For this review, take the finished solid that the model builds, in its own axes (mm). A direction names the side the tool comes from. Give positions to 0.01 mm unless a question says otherwise; leave off trailing zeros. Write each loop counter-clockwise with the first axis right and the second up, starting at its lowest first coordinate (ties: lowest second). Pieces come first, ordered by that corner, then holes. Notation, with made-up numbers: (-20.75, -4.5) -> (2.25, -4.5) arc R16 ccw to (2.25, 22.5) -> close; hole circle Ø7 at (-21, -38.5). An arc over 180 degrees is marked (long way). Write item = value, one per line.
```python
from build123d import *

# Parameters (mm, degrees)
F0_W     = 88
F0_H     = 30
F1_DEPTH = 5
F2_R     = 4
F3_DEPTH = 8
F4_R     = 4
F5_DEPTH = 8


with BuildPart() as f1:
    # F0 (on Front) → F1 (new body)
    with BuildSketch(Plane.XZ):
        Rectangle(F0_W, F0_H)
    extrude(amount=F1_DEPTH)

    # F2 (on face) → F3 (join)
    with BuildSketch(Plane.XZ.offset(5)):
        with Locations((-29, 0)):
            Circle(F2_R)
    extrude(amount=F3_DEPTH)

    # F4 (on face) → F5 (join)
    with BuildSketch(Plane.XZ.offset(5)):
        Circle(F4_R)
        with Locations((25, 0)):
            Circle(F4_R)
    extrude(amount=F5_DEPTH)


solid = f1.part
```
(1) To check wall thickness, follow probe 1 along Y at (x, z) = (3, 4.5); probe 2 along X at (y, z) = (-6, -3.5); probe 3 along X at (y, z) = (-6.75, 3). State the ranges of each line that lie inside material, in increasing order.
Answers below:
probe_1 = -5 to 0
probe_2 = -30.94 to -27.06, -1.94 to 1.94, 23.06 to 26.94
probe_3 = -31.65 to -26.35, -2.65 to 2.65, 22.35 to 27.65
(2) The part is to be moulded in two halves that separate along X. For faces 1 (the face through (-1, 0, 0)), 2 (the face through (-0.867, -8.944, -3.905)), 3 (the face through (-32.2, -8.9, -2.4)), 4 (the face through (-44, -2, 0)), say which applies: released by +X, released by -X, zero draft, split by the parting line, or undercut.
Answers below:
face_1 = zero draft
face_2 = undercut
face_3 = undercut
face_4 = released by -X
(3) Tool access review of faces 5 (the face through (-1, -2, 15)), 6 (the face through (-1, -5, 7)): name each direction out of +Z, -Z, +X, -X, +Y, -Y from which nothing blocks a thin tool from reaching the whole face with its end or side.
Answers below:
face_5 = +Z, +X, -X, +Y, -Y
face_6 = -Y
(4) Take a section at B-B (y = -8.75). Write out the cut boundary in (x, z).
Answers below:
outline = circle Ø8 at (-29, 0); circle Ø8 at (0, 0); circle Ø8 at (25, 0)
(5) Take a section at A-A (x = 0). Write out the cut boundary in (y, z), plus the area to 3 significant figures.
Answers below:
outline = (-13, -4) -> (-5, -4) -> (-5, -15) -> (0, -15) -> (0, 15) -> (-5, 15) -> (-5, 4) -> (-13, 4) -> close
area = 214 mm^2
(6) Take a section at C-C (z = 0). Write out the cut boundary in (x, y), plus the area to 3 significant figures.
Answers below:
outline = (-44, -5) -> (-33, -5) -> (-33, -13) -> (-25, -13) -> (-25, -5) -> (-4, -5) -> (-4, -13) -> (4, -13) -> (4, -5) -> (21, -5) -> (21, -13) -> (29, -13) -> (29, -5) -> (44, -5) -> (44, 0) -> (-44, 0) -> close
area = 632 mm^2
(7) For pin 1 (1 mm diameter, centred on x = -10.5, z = -6.5, fed in from -Y), flat-tipped, find the tip position at first contact; note if it passes through.
Answers below:
pin_1 = -5
(8) Take a section at D-D (x = -27). Write out the cut boundary in (y, z), plus the area to 3 significant figures.
Answers below:
outline = (-13, -3.46) -> (-5, -3.46) -> (-5, -15) -> (0, -15) -> (0, 15) -> (-5, 15) -> (-5, 3.46) -> (-13, 3.46) -> close
area = 205 mm^2
